Autodesk Inventor part; units mm, degrees
ref_plane "YZ Plane" through (0, 0, 0) normal (1, 0, 0) x (0, 1, 0)
ref_plane "XZ Plane" through (0, 0, 0) normal (0, 1, 0) x (-1, 0, 0)
ref_plane "XY Plane" through (0, 0, 0) normal (0, 0, 1) x (1, 0, 0)
sketch "草图1" plane through (0, 0, 0) normal (0, 0, 1) x (1, 0, 0)
  circle A0 centre (0, 0) radius 20
  circle A1 centre (0, 0) radius 35
  line L0 (-35, 0) -> (35, 0)
  point P0 (-20, 0)
  point P1 (20, 0)
  dimension "d0" = 70
  dimension "d1" = 70
extrude "拉伸1" add sketch "草图1" along normal mid plane 20 contours A0 L0 A1 picked at (29.7075, 2.5961)
sketch "草图2" plane through (0, 0, 0) normal (0, 0, 1) x (1, 0, 0)
  arc A0 (20, 0) -> (-20, 0) centre (0, 0) ccw
  line L0 (-20, 0) -> (-40, 0)
  line L1 (-40, 0) -> (-40, 10)
  line L2 (-40, 10) -> (-20, 10)
  line L3 (-20, 10) -> (-20, 0)
  line L4 (35, 0) -> (20, 0)
  line L5 (20, 0) -> (40, 0)
  line L6 (40, 0) -> (40, 10)
  line L7 (40, 10) -> (20, 10)
  line L8 (20, 10) -> (20, 0)
  dimension "d4" = 20
  dimension "d5" = 10
  dimension "d6" = 20
  dimension "d7" = 10
extrude "拉伸2" add sketch "草图2" along normal mid plane 30
sketch "草图3" plane through (0, 0, 0) normal (0, 0, 1) x (1, 0, 0)
  circle A0 centre (0, 150) radius 15
  line L0 (-20, 10) -> (-33.541, 10)
  arc A1 (33.541, 10) -> (-33.541, 10) centre (0, 0) ccw
  line L1 (33.541, 10) -> (20, 10)
  line L2 (20, 10) -> (20, 0)
  arc A2 (20, 0) -> (-20, 0) centre (0, 0) ccw
  line L3 (-20, 0) -> (-20, 10)
  circle A3 centre (0, 0) radius 35
  line L4 (-14.8661, 152) -> (-34.6875, 4.6667)
  line L5 (0, 0) -> (0, 98.8257)
  line L6 (14.8661, 152) -> (34.6875, 4.6667)
  dimension "d10" = 30
  dimension "d11" = 150
extrude "拉伸3" add sketch "草图3" along normal mid plane 20 contours A0 | A0 L6 A3 A1 L4
sketch "草图4" plane through (0, 0, 10) normal (0, 0, 1) x (1, 0, 0)
  arc A0 (14.8661, 152) -> (-14.8661, 152) centre (0, 150) ccw
  point P0 (0, 0)
hole "孔1" at (0, 150, 10) direction (0, 0, -1) diameter 10 end through all
sketch "草图5" plane through (-40, 0, 15) normal (0, -1, 0) x (1, 0, 0)
  line L0 (20, -5) -> (20, 0) construction
  line L1 (0, 0) -> (20, 0) construction
  line L2 (0, -30) -> (0, 0) construction
  line L3 (20, -30) -> (0, -30) construction
  line L4 (20, -30) -> (20, -25) construction
  line L5 (20, -5) -> (20, -25) construction
  point P0 (40, -15)
  point P1 (10, -15)
  point P2 (0, -15)
  point P3 (10, -30)
hole "孔2" at (-30, 0, 0) direction (0, 1, 0) diameter 10 end through all
mirror "镜像1" about plane through (0, 0, 0) normal (1, 0, 0) of "孔2"
properties part number "连杆"
Could you check a few things on this model? Use its own coordinates, in mm. A direction names the side the tool comes from. Coordinates: 2 decimals unless noted, no trailing zeros. Order: outer loops, then holes, each group sorted by start corner. A loop starts at its lowest first (then second) coordinate and runs counter-clockwise, first axis right, second up. Notation, with made-up numbers: M -29.5,-16 L 2.5,-16 A22 cw 2.5,14 Z; hole C 15.5,-30.5 d5. An arc over 180 degrees is marked long. Use a Markdown table: item, result. Add a question column.
Q1. I want a section at B-B on z = -1.25. List the corners of the cut face in (x, y) for me, then the cut area to 3 significant figures.
Q2. I want a section at A-A on z = -11.75. List the corners of the cut face in (x, y) for me, then the cut area to 3 significant figures.
Q3. I want a section at C-C on y = 150. List the corners of the cut face in (x, z) for me, then the cut area to 3 significant figures.
Q4. I'm going to push flat-ended pins straight in: pin 1 (16 mm diameter, centred on x = 0, y = 150, fed in from -Z); pin 2 (4 mm diameter, centred on y = 70.5, z = -3, fed in from +X); pin 3 (20.5 mm diameter, centred on x = 9.5, y = 48, fed in from +Z); pin 4 (2 mm diameter, centred on x = 32, z = 10.5, fed in from -Y). Where does each tip first touch, or does it pass through?
Q5. Which directions (+Z, -Z, +X, -X, +Y, -Y) give clear straight access to the entire face, cutting with the end or side of a thin tool? Please do faces 1 (the flat face through (35, 10, -4)), 2 (the flat face through (40, 5, 0)), 3 (the flat face through (-20, 5, 12)), 4 (the flat face through (-20, 5, -13)).
Q6. I want a section at D-D on x = 27.5. List the corners of the cut face in (y, z) for me, then the cut area to 3 significant figures.
Q7. We'd pull the mould along X, two halves only. Please class faces 5 (the flat face through (22.16, 97.77, -0.14)), 6 (the flat face through (20, 5, 12)), 7 (the flat face through (30, 5, 15)): pulls with the +X half, pulls with the -X half, needs draft (parallel to the pull), parting line crosses it, or undercut.
Q8. If I drill on L1, parallel to X at y = 33.5, z = 0; L2, parallel to Z at x = 23.5, y = 17; L3, parallel to Y at x = 35, z = -10.25, over which ranges is the centre line in solid material (lowest first)?
Checked values:
| question | item | result |
|---|---|---|
| 1 | outline | M -40,0 L -34.84,0 L -34.84,10 L -40,10 Z; M -25.16,0 L -20,0 A20 cw 20,0 L 25.16,0 L 25.16,75.49 L 14.87,152 A15 ccw -14.87,152 L -25.16,75.49 Z; M 34.84,0 L 40,0 L 40,10 L 34.84,10 Z; hole C 0,150 d10 |
| 1 | area | 6,550 mm² |
| 2 | outline | M -40,0 L -20,0 L -20,10 L -40,10 Z; M 20,0 L 40,0 L 40,10 L 20,10 Z |
| 2 | area | 400 mm² |
| 3 | outline | M -15.14,-10 L -5,-10 L -5,10 L -15.14,10 Z; M 5,-10 L 15.14,-10 L 15.14,10 L 5,10 Z |
| 3 | area | 405 mm² |
| 4 | pin 1 | z = -10 |
| 4 | pin 2 | x = 26.1 |
| 4 | pin 3 | z = 10 |
| 4 | pin 4 | y = 0 |
| 5 | face 1 | +X, +Y |
| 5 | face 2 | +Z, -Z, +X, +Y, -Y |
| 5 | face 3 | +Z, +Y, -Y |
| 5 | face 4 | -Z, +Y, -Y |
| 6 | outline | M 0,-15 L 10,-15 L 10,-10 L 58.09,-10 L 58.09,-4.33 L 0,-4.33 Z; M 0,4.33 L 58.09,4.33 L 58.09,10 L 10,10 L 10,15 L 0,15 Z |
| 6 | area | 759 mm² |
| 7 | face 5 | pulls with the +X half |
| 7 | face 6 | undercut |
| 7 | face 7 | needs draft |
| 8 | L1 | -25 to 25 |
| 8 | L2 | -10 to 10 |
| 8 | L3 | 0 to 10 |
